The listing builds one solid part. Answer for the finished solid, in the listing's coordinates (mm). Face numbers are marked on the shaded views. A direction names the side the tool comes from. Round coordinates to 2 decimals unless told otherwise and drop trailing zeros. Write each loop counter-clockwise with the first axis right and the second up, starting at its lowest first coordinate (ties: lowest second). Pieces come first, ordered by that corner, then holes.
Item 1: Find section A-A on y = -10.5. Give the vertices of the cut face in (x, z), then the cut area to 3 significant figures.
Item 2: Each of these flat-tipped pins is pushed along its axis until it touches: pin 1 (6 mm diameter, centred on x = -16.5, z = 3.5, fed in from -Y); pin 2 (5.5 mm diameter, centred on y = 5.5, z = -41, fed in from +X); pin 3 (8.5 mm diameter, centred on y = 4.5, z = 3.5, fed in from -X). Where does it stop, or does it pass through?
Item 3: A tool of negligible diameter and unlimited length cuts with its end or side. For the marked faces 1 and 2, from which of +Z, -Z, +X, -X, +Y, -Y can it reach the whole face along a straight path? Write none if from no direction.
Item 4: Find section C-C on z = -26. Give the vertices of the cut face in (x, y).
Item 5: Find section B-B on y = 0. Give the vertices of the cut face in (x, z), then the cut area to 3 significant figures.
Item 6: Find the intervals of material crossed by probe 1 along Z at (x, y) = (-42, -1); probe 2 along X at (y, z) = (-0.5, -36.5); probe 3 along Z at (x, y) = (-18.5, 13.5), in increasing order.
Item 7: Find section D-D on y = -16. Give the vertices of the cut face in (x, z), then the cut area to 3 significant figures.
Item 8: For a pull along Z with two mould halves and no side action, classify the marked faces 3, 4 and 5 as +Z half, -Z half, draft (parallel to the pull), parting line (faces both ways), or undercut.
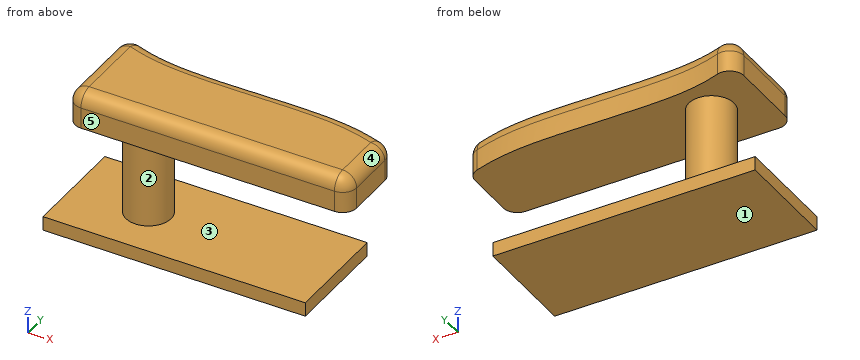
```python
from build123d import *

# Parameters (mm, degrees)
F0_W     = 101.6
F0_H     = 38.1
F1_DEPTH = 12.7
F3_DEPTH = 25.4
F4_R     = 5.08
F5_R     = 8.1585403427
F6_DEPTH = 38.1
F7_W     = 94.6341231465
F7_H     = 38.4192988276
F8_DEPTH = 5.08


# Not quite as in the source:
# - two fillets or chamfers of one size are made in one step


with BuildPart() as f1:
    # F0 (on Top) → F1 (new body)
    with BuildSketch(Plane.XY):
        Rectangle(F0_W, F0_H)
    extrude(amount=F1_DEPTH)

    # F2 (on face) → F3 (cut)
    with BuildSketch(Plane.XY.offset(12.7)):
        with BuildLine():
            Line((-50.8, 29.4957049191), (-50.8, 19.05))
            add(Edge.make_bspline(
                [(-50.8, 19.05), (-44.8058190597, 16.5548569949), (-29.3022913601, 10.1013449841), (28.5345191575, 14.5340371651), (44.5678818935, 9.2526124329), (50.8, 7.199739106)],
                knots=[0, 0, 0, 0, 0.2781516974, 0.7194198154, 1, 1, 1, 1], degree=3))
            Line((50.8, 7.199739106), (51.4432899654, 29.4957049191))
            Line((51.4432899654, 29.4957049191), (-50.8, 29.4957049191))
        make_face()
    extrude(amount=-F3_DEPTH, mode=Mode.SUBTRACT)

    # F4
    f4_edges = [f1.edges().sort_by_distance(p)[0] for p in [
        (0, -19.05, 12.7),
        (50.8, -5.92513, 12.7),
        (-0.16927, 12.372824, 12.7),
        (-50.8, 0, 12.7),
        (-50.8, 19.05, 6.35),
        (-50.8, -19.05, 6.35),
        (50.8, 7.199739, 6.35),
        (50.8, -19.05, 6.35),
    ]]
    fillet(f4_edges, radius=F4_R)

    # F5 (on Top) → F6 (join)
    with BuildSketch(Plane.XY):
        with Locations((-32.3988236487, 0)):
            Circle(F5_R)
    extrude(amount=-F6_DEPTH)

    # F7 (on face) → F8 (join)
    with BuildSketch(Plane(origin=(0, 0, -38.1), x_dir=(1, 0, 0), z_dir=(0, 0, -1))):
        with Locations((-12.0352953672, -0.0617783517)):
            Rectangle(F7_W, F7_H)
    extrude(amount=F8_DEPTH)


solid = f1.part
```
Check values:
1. outline: (-59.35, -43.18) - (35.28, -43.18) - (35.28, -38.1) - (-59.35, -38.1) - close; (-50.8, 0) - (50.8, 0) - (50.8, 7.62) arc R5.08 ccw to (45.72, 12.7) - (-45.72, 12.7) arc R5.08 ccw to (-50.8, 7.62) - close
1. area: 1,760 mm2
2. pin 1: stops at y = -19.05
2. pin 2: stops at x = 35.28
2. pin 3: stops at x = -50.8
3. face 1: -Z, +X, -X, +Y, -Y
3. face 2: none
4. outline: circle Ø16.32 at (-32.4, 0)
5. outline: (-59.35, -43.18) - (35.28, -43.18) - (35.28, -38.1) - (-24.24, -38.1) - (-24.24, 0) - (50.8, 0) - (50.8, 7.62) arc R5.08 ccw to (45.72, 12.7) - (-45.72, 12.7) arc R5.08 ccw to (-50.8, 7.62) - (-50.8, 0) - (-40.56, 0) - (-40.56, -38.1) - (-59.35, -38.1) - close
5. area: 2,380 mm2
6. probe 1: z = -43.18 to -38.1, 0 to 12.7
6. probe 2: x = -40.54 to -24.26
6. probe 3: z = -43.18 to -38.1
7. outline: (-59.35, -43.18) - (35.28, -43.18) - (35.28, -38.1) - (-59.35, -38.1) - close; (-50.38, 0) - (50.38, 0) - (50.38, 7.62) arc R4.66 ccw to (45.72, 12.28) - (-45.72, 12.28) arc R4.66 ccw to (-50.38, 7.62) - close
7. area: 1,710 mm2
8. face 3: undercut
8. face 4: +Z half
8. face 5: draft
